The listing builds one solid part. Answer for the finished solid, in the listing's coordinates (mm). A direction names the side the tool comes from. Coordinates: 2 decimals unless noted, no trailing zeros. Loops run counter-clockwise (first coordinate to the right, second up) from the corner with the lowest first, then second, coordinate; pieces in that order, holes last. Notation, with made-up numbers: (83, 36) - (100, 36) arc R7 cw to (100, 48) - close; hole circle Ø6 at (63, 44.5). An arc over 180 degrees is marked (long way). Put each result on its own line as item: value.
```python
from build123d import *

# Parameters (mm, degrees)
SKETCH1_W           = 3.175
SKETCH1_H           = 47.625
SKETCH1_W_2         = 25.4
SKETCH1_H_2         = 3.175
BOSS_EXTRUDE1_DEPTH = 30.48
SKETCH2_R           = 5.08
CUT_EXTRUDE1_DEPTH  = 32.766
SKETCH3_R           = 2.4892
CUT_EXTRUDE2_DEPTH  = 32.766


with BuildPart() as part:
    # Sketch1 → Boss-Extrude1 (new body)
    with BuildSketch(Plane(origin=(0, 0, 0), x_dir=(1, 0, 0), z_dir=(0, 1, 0))):
        with Locations((1.5875, 23.8125)):
            Rectangle(SKETCH1_W, SKETCH1_H)
        with Locations((15.875, 49.2125)):
            Rectangle(SKETCH1_W_2, SKETCH1_H_2)
        with Locations((1.5875, 49.2125)):
            Rectangle(SKETCH1_W, SKETCH1_H_2)
    extrude(amount=BOSS_EXTRUDE1_DEPTH)

    # Sketch2 → Cut-Extrude1 (cut)
    with BuildSketch(Plane.XY.offset(-47.625)):
        with Locations((19.05, 15.24)):
            Circle(SKETCH2_R)
    extrude(amount=-CUT_EXTRUDE1_DEPTH, mode=Mode.SUBTRACT)

    # Sketch3 → Cut-Extrude2 (cut)
    with BuildSketch(Plane(origin=(3.175, 0, 0), x_dir=(0, 0, -1), z_dir=(1, 0, 0))):
        with Locations((12.7, 15.24)):
            Circle(SKETCH3_R)
        with Locations((25.4, 15.24)):
            Circle(SKETCH3_R)
        with Locations((38.1, 15.24)):
            Circle(SKETCH3_R)
    extrude(amount=-CUT_EXTRUDE2_DEPTH, mode=Mode.SUBTRACT)


solid = part.part
```
1) For a pull along Y with two mould halves and no side action, classify faces 1 (the face through (15.02, 12.15, -49.19)), 2 (the face through (3, 30.48, -33)), 3 (the face through (11, 15, -50.8)) as pulls with the +Y half, pulls with the -Y half, needs draft (parallel to the pull), parting line crosses it, or undercut.
Found:
face 1: undercut
face 2: pulls with the +Y half
face 3: needs draft
2) Each of these flat-tipped pins is pushed along its axis until it touches: pin 1 (9 mm diameter, centred on y = 20, z = -28, fed in from +X) (3 decimals); pin 2 (13 mm diameter, centred on x = 19.05, y = 15.24, fed in from +Z) (3 decimals). Where does it stop, or does it pass through?
Found:
pin 1: stops at x = 3.175
pin 2: stops at z = -47.625
3) The part is cut by section C-C (y = 15.24). Give the vertices of the cut face in (x, z) (3 decimals).
Found:
outline: (0, -50.8) - (13.97, -50.8) - (13.97, -47.625) - (3.175, -47.625) - (3.175, -40.589) - (0, -40.589) - close; (0, -35.611) - (3.175, -35.611) - (3.175, -27.889) - (0, -27.889) - close; (0, -22.911) - (3.175, -22.911) - (3.175, -15.189) - (0, -15.189) - close; (0, -10.211) - (3.175, -10.211) - (3.175, 0) - (0, 0) - close; (24.13, -50.8) - (28.575, -50.8) - (28.575, -47.625) - (24.13, -47.625) - close
4) The part is cut by section B-B (z = -25.4). Give the vertices of the cut face in (x, y) (3 decimals), and give its area (3 significant figures).
Found:
outline: (0, 0) - (3.175, 0) - (3.175, 12.751) - (0, 12.751) - close; (0, 17.729) - (3.175, 17.729) - (3.175, 30.48) - (0, 30.48) - close
area: 81.0 mm^2
5) The part is cut by section D-D (y = 26). Give the vertices of the cut face in (x, z) (3 decimals), and give its area (3 significant figures).
Found:
outline: (0, -50.8) - (28.575, -50.8) - (28.575, -47.625) - (3.175, -47.625) - (3.175, 0) - (0, 0) - close
area: 242 mm^2
6) For faces 4 (the face through (13, 15, -47.625)), 5 (the face through (1.61, 15.349, -35.613)), determine the directions among +Z, -Z, +X, -X, +Y, -Y from which every point of the face is accessible in a straight line to the end or side of a thin tool.
Found:
face 4: +Z, +X, +Y, -Y
face 5: +X, -X
7) The part is cut by section A-A (x = 19.05). Give the vertices of the cut face in (y, z) (3 decimals).
Found:
outline: (0, -50.8) - (10.16, -50.8) - (10.16, -47.625) - (0, -47.625) - close; (20.32, -50.8) - (30.48, -50.8) - (30.48, -47.625) - (20.32, -47.625) - close
8) Straight lines are drawn through the part: L1, parallel to Y at x = 1.4, z = -25.4; L2, parallel to X at y = 15, z = -48 (3 decimals); L3, parallel to X at y = 28, z = -31.5 (3 decimals). For each, find the intervals that lie inside material, in ascending order. Write a range as [from, to].
Found:
L1: y = [0, 12.75], [17.73, 30.48]
L2: x = [0, 13.976], [24.124, 28.575]
L3: x = [0, 3.175]
